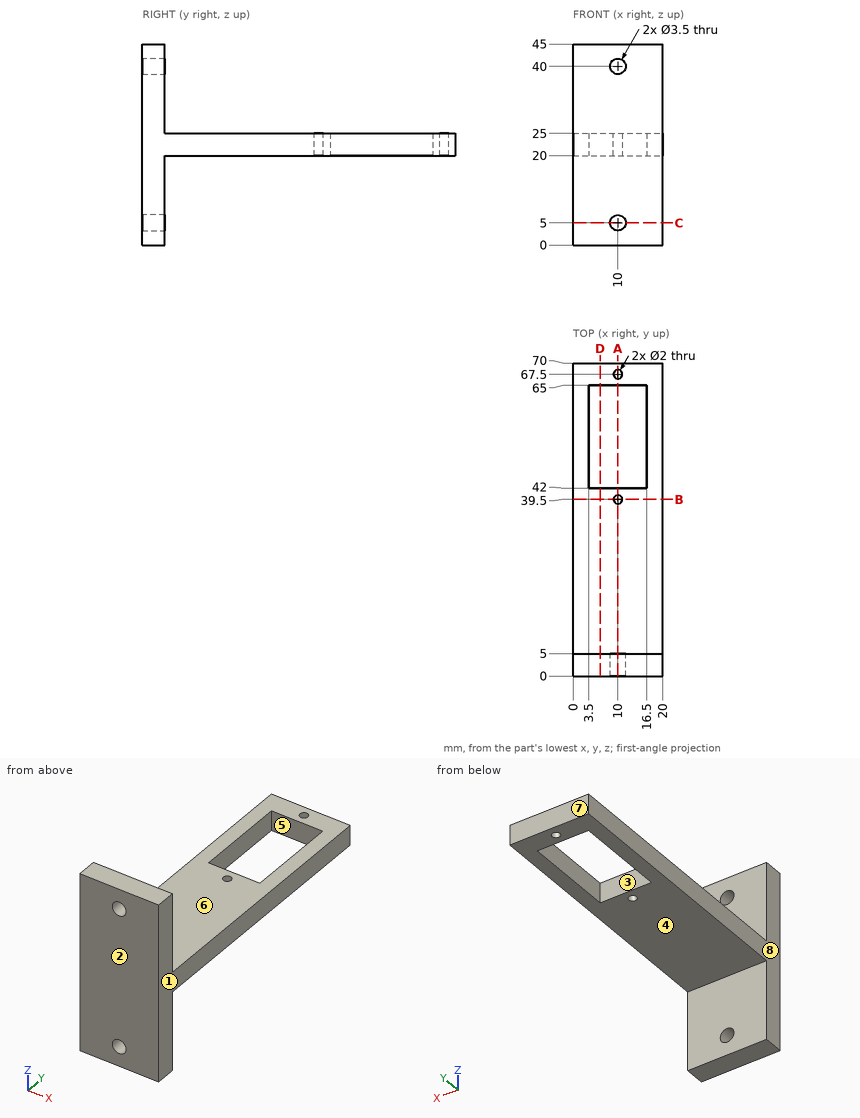
Study the drawing (mm; zero at the part's minimum x, y, z) and answer. A direction names the side the tool comes from. Coordinates: 2 decimals unless noted, no trailing zeros. Loops run counter-clockwise (first coordinate to the right, second up) from the corner with the lowest first, then second, coordinate; pieces in that order, holes last. Notation, with made-up numbers: M 83.25,41.25 L 107.25,41.25 A19 cw 107.25,58.25 Z; hole C -20,-39.75 d8. An arc over 180 degrees is marked long. Answer in a Markdown table with one row per item. Add a question column.
1. Find section B-B, the plane y = 39.5. Write down the section's boundary in (x, z).
2. The mould has two halves that part along Y. Classify the marked faces 1, 2 and 3: pulls with the +Y half, pulls with the -Y half, needs draft (parallel to the pull), parting line crosses it, or undercut.
3. Find section C-C, the plane z = 5. Write down the section's boundary in (x, y), then the cut area to 3 significant figures.
4. Find section D-D, the plane x = 6. Write down the section's boundary in (y, z).
5. A tool of negligible diameter and unlimited length cuts with its end or side. For the marked faces 4, 5, 6, 7 and 8, from which of +Z, -Z, +X, -X, +Y, -Y can it reach the whole face along a straight path? Write none if from no direction.
6. Flat-ended cylindrical pins translate along their axes: P1, Ø6, axis at x = 13.5, z = 11, coming from the +Y side; P2, Ø5, axis at x = 6.5, y = 57.5, coming from the -Z side; P3, Ø2.5, axis at x = 10, y = 67.5, coming from the -Z side; P4, Ø2, axis at x = 4.5, y = 9.5, coming from the +Z side. Find the tip coordinate at first contact, or state that the pin passes through.
7. Find section A-A, the plane x = 10. Write down the section's boundary in (y, z).
8. Consider L1, parallel to X at y = 1, z = 5; L2, parallel to X at y = 67.5, z = 23.25; L3, parallel to Y at x = 6.25, z = 39.5. Determine where each line is inside the solid, lowest interval first.
Reported:
| question | item | result |
|---|---|---|
| 1 | outline | M 0,20 L 9,20 L 9,25 L 0,25 Z; M 11,20 L 20,20 L 20,25 L 11,25 Z |
| 2 | face 1 | needs draft |
| 2 | face 2 | pulls with the -Y half |
| 2 | face 3 | undercut |
| 3 | outline | M 0,0 L 8.25,0 L 8.25,5 L 0,5 Z; M 11.75,0 L 20,0 L 20,5 L 11.75,5 Z |
| 3 | area | 82.5 mm^2 |
| 4 | outline | M 0,0 L 5,0 L 5,20 L 42,20 L 42,25 L 5,25 L 5,45 L 0,45 Z; M 65,20 L 70,20 L 70,25 L 65,25 Z |
| 5 | face 4 | -Z, +X, -X, +Y |
| 5 | face 5 | +Z, -Z |
| 5 | face 6 | +Z, +X, -X, +Y |
| 5 | face 7 | +Z, -Z, +X, -X, +Y |
| 5 | face 8 | +Z, -Z, -X, +Y, -Y |
| 6 | P1 | stops at y = 5 |
| 6 | P2 | passes through |
| 6 | P3 | stops at z = 20 |
| 6 | P4 | stops at z = 25 |
| 7 | outline | M 0,0 L 5,0 L 5,3.25 L 0,3.25 Z; M 0,6.75 L 5,6.75 L 5,20 L 38.5,20 L 38.5,25 L 5,25 L 5,38.25 L 0,38.25 Z; M 0,41.75 L 5,41.75 L 5,45 L 0,45 Z; M 40.5,20 L 42,20 L 42,25 L 40.5,25 Z; M 65,20 L 66.5,20 L 66.5,25 L 65,25 Z; M 68.5,20 L 70,20 L 70,25 L 68.5,25 Z |
| 8 | L1 | x = 0 to 8.25, 11.75 to 20 |
| 8 | L2 | x = 0 to 9, 11 to 20 |
| 8 | L3 | y = 0 to 5 |
